For this review, take the finished solid that the model builds, in its own axes (mm). A direction names the side the tool comes from. Give positions to 0.01 mm unless a question says otherwise; leave off trailing zeros. Write each loop counter-clockwise with the first axis right and the second up, starting at its lowest first coordinate (ties: lowest second). Pieces come first, ordered by that corner, then holes.
Q1. Insertion check: P1, Ø4, axis at x = -8, y = 24, coming from the -Z side; P2, Ø1.6, axis at y = 0.5, z = 1.5, coming from the +X side. Each pin has a flat end and moves straight along its axis. Give the tip position at first contact, or say it passes through.
Q2. Machinability: for faces 1 (the flat face through (-19, 2.73, 3)), 2 (the flat face through (0, 13, 5.461)), 3 (the flat face through (19, 2.73, 3)), which of the approach directions +Z, -Z, +X, -X, +Y, -Y give a long, thin tool a straight path to every point of the face, cutting with its end or side? Answer none if there is none.
Q3. For line 1 (X direction, y = 1, z = 2.7); line 2 (Y direction, x = -13, z = 1), list the stretches that pass through material, from the lowest coordinate up.
Q4. We need section A-A (z = 1.5). Write out the cut boundary in (x, y), then the cut area to 3 significant figures.
Q5. We need section B-B (x = 21). Write out the cut boundary in (y, z).
```python
from build123d import *

# Parameters (mm, degrees)
SKETCH1_W           = 25.4
SKETCH1_H           = 5.461
BOSS_EXTRUDE1_DEPTH = 5.461


with BuildPart() as part:
    # Sketch1 → Boss-Extrude1 (new body)
    with BuildSketch(Plane.XY):
        Polygon((-25.4, 2.7305), (-12.7, 2.7305), (12.7, 2.7305), (25.4, 2.7305), (25.4, 27.3685), (-25.4, 27.3685), align=None)
        Rectangle(SKETCH1_W, SKETCH1_H)
    extrude(amount=BOSS_EXTRUDE1_DEPTH)


solid = part.part
```
Computed:
1. P1: stops at z = 0
1. P2: stops at x = 12.7
2. face 1: +Z, -Z, -X, -Y
2. face 2: +Z, +X, -X, +Y, -Y
2. face 3: +Z, -Z, +X, -Y
3. line 1: x = -12.7 to 12.7
3. line 2: y = 2.73 to 27.37
4. outline: (-25.4, 2.73) - (-12.7, 2.73) - (-12.7, -2.73) - (12.7, -2.73) - (12.7, 2.73) - (25.4, 2.73) - (25.4, 27.37) - (-25.4, 27.37) - close
4. area: 1,390 mm2
5. outline: (2.73, 0) - (27.37, 0) - (27.37, 5.46) - (2.73, 5.46) - close
